Could you check a few things on this model? Use its own coordinates, in mm. A direction names the side the tool comes from. Round coordinates to 2 decimals unless told otherwise and drop trailing zeros. Loops run counter-clockwise (first coordinate to the right, second up) from the corner with the lowest first, then second, coordinate; pieces in that order, holes last. Notation, with made-up numbers: M 47.25,32.5 L 58.25,32.5 A16 cw 58.25,36.5 Z; hole C 28,54.5 d5. An arc over 180 degrees is marked long. One line per item, written item: value. Start each with the question number.
Q1. I'm going to push flat-ended pins straight in: pin 1 Ø1.8 at (y, z) = (24.5, 5.5) entering from -X; pin 2 Ø11 at (y, z) = (9.5, 107.5) entering from -X; pin 3 Ø5 at (x, z) = (19.5, 106.5) entering from +Y; pin 4 Ø6 at (x, y) = (23, -36.5) entering from +Z. Where does each tip first touch, or does it pass through?
Q2. Which directions (+Z, -Z, +X, -X, +Y, -Y) give clear straight access to the entire face, cutting with the end or side of a thin tool? Please do faces 4 (the face through (19.38, 23.7, 21.69)), 5 (the face through (3.711, -43.335, 14.252)), 6 (the face through (19.199, 19.981, 92.714)), 7 (the face through (28.813, 22, 52)), 8 (the face through (27.2, 19.51, 101.73)).
Q3. Imagine slicing it at A-A (y = 11.5). Please give me the cut outline in (x, z).
Q4. Please list where these lines run through material, in increasing order: line 1 along X through (y, z) = (-44, 18); line 2 along Z through (x, y) = (10.5, -24.5); line 3 along X through (y, z) = (23, 55.5).
Q5. Thinking about a two-plate mould opening in Y: for faces 1 (the face through (9.73, -39.325, 59.103)), 2 (the face through (9.763, 22, 50)), 3 (the face through (19.38, 23.97, 16.62)), which applies, released by +Y, released by -Y, zero draft, split by the parting line, or undercut?
Q6. Imagine slicing it at B-B (z = 29). Please give me the cut outline in (x, y), then the cut area to 3 significant figures.
Q7. Imagine slicing it at D-D (y = 0.5). Please give me the cut outline in (x, z).
Q8. Imagine slicing it at C-C (x = 2). Please give me the cut outline in (y, z).
from build123d import *

# Parameters (mm, degrees)
F0_W     = 63.5
F0_H     = 63.5
F1_DEPTH = 101.6
F1_TAPER = 3
F3_DEPTH = 10.16
F4_W     = 7.62
F4_H     = 7.62
F5_DEPTH = 7.62
F5_TAPER = 26
F7_DEPTH = 2.54
F8_W     = 12.7
F8_H     = 12.7
F9_DEPTH = 5.08


with BuildPart() as f1:
    # F0 (on Top) → F1 (new body)
    with BuildSketch(Plane.XY):
        with Locations((3.6575980484, -9.4182148212)):
            Rectangle(F0_W, F0_H)
    extrude(amount=F1_DEPTH, taper=F1_TAPER)

    # F2 (on face) → F3 (join)
    with BuildSketch(Plane.XY.offset(101.6)):
        Polygon((-12.6077715764, -15.5235844461), (-22.7677715764, -15.5235844461), (-22.7677715764, -35.8435844461), (-12.6077715764, -35.8435844461), (-2.4477715764, -35.8435844461), (-2.4477715764, -25.6835844461), (-12.6077715764, -25.6835844461), align=None)
        Polygon((19.9229676733, -35.8435844461), (30.0829676733, -35.8435844461), (30.0829676733, -15.5235844461), (19.9229676733, -15.5235844461), (19.9229676733, -25.6835844461), (9.7629676733, -25.6835844461), (9.7629676733, -35.8435844461), align=None)
        Polygon((-12.6077715764, 17.0071548036), (-22.7677715764, 17.0071548036), (-22.7677715764, -3.3128451964), (-12.6077715764, -3.3128451964), (-12.6077715764, 6.8471548036), (-2.4477715764, 6.8471548036), (-2.4477715764, 17.0071548036), align=None)
        Polygon((30.0829676733, -3.3128451964), (30.0829676733, 17.0071548036), (19.9229676733, 17.0071548036), (9.7629676733, 17.0071548036), (9.7629676733, 6.8471548036), (19.9229676733, 6.8471548036), (19.9229676733, -3.3128451964), align=None)
    extrude(amount=F3_DEPTH)

    # F4 (on face) → F5 (join)
    with BuildSketch(Plane(origin=(0, -41.0554529271, 2.1516251154), x_dir=(1, 0, 0), z_dir=(0, -0.9986295348, 0.0523359562))):
        with Locations((-19.2024019516, 14.3554221105)):
            Rectangle(F4_W, F4_H)
        with Locations((3.6575980484, 14.3554221105)):
            Rectangle(F4_W, F4_H)
        with Locations((26.5175980484, 14.3554221105)):
            Rectangle(F4_W, F4_H)
    extrude(amount=F5_DEPTH, taper=F5_TAPER)

    # F6 (on face) → F7 (join)
    with BuildSketch(Plane(origin=(0, -41.0554529271, 2.1516251154), x_dir=(1, 0, 0), z_dir=(0, -0.9986295348, 0.0523359562))):
        Polygon((-11.5824019516, 56.964216193), (-11.5824019516, 41.724216193), (18.8975980484, 41.724216193), (18.8975980484, 56.964216193), (18.8975980484, 62.044216193), (12.5475980484, 62.044216193), (12.5475980484, 56.964216193), (6.8325980484, 56.964216193), (6.8325980484, 62.044216193), (0.4825980484, 62.044216193), (0.4825980484, 56.964216193), (-5.2324019516, 56.964216193), (-5.2324019516, 62.044216193), (-11.5824019516, 62.044216193), align=None)
    extrude(amount=F7_DEPTH)

    # F8 (on face) → F9 (join)
    with BuildSketch(Plane(origin=(0, 22.2706172509, 1.1671535934), x_dir=(-1, 0, 0), z_dir=(0, 0.9986295348, 0.0523359562))):
        Polygon((-28.8129676733, 100.5706750214), (-28.8129676733, -1.1687553319), (-25.6379676733, -1.1687553319), (-25.6379676733, 15.3412446681), (-12.9379676733, 15.3412446681), (-12.9379676733, -1.1687553319), (-9.7629676733, -1.1687553319), (-9.7629676733, 100.5706750214), (-12.9379676733, 100.5706750214), (-12.9379676733, 91.5412446681), (-25.6379676733, 91.5412446681), (-25.6379676733, 100.5706750214), align=None)
        with Locations((-19.2879676733, 26.7712446681)):
            Rectangle(F8_W, F8_H, mode=Mode.SUBTRACT)
        with Locations((-19.2879676733, 44.5512446681)):
            Rectangle(F8_W, F8_H, mode=Mode.SUBTRACT)
        with Locations((-19.2879676733, 80.1112446681)):
            Rectangle(F8_W, F8_H, mode=Mode.SUBTRACT)
        with Locations((-19.2879676733, 62.3312446681)):
            Rectangle(F8_W, F8_H, mode=Mode.SUBTRACT)
    extrude(amount=F9_DEPTH)


solid = f1.part
Report:
1. pin 1: stops at x = 9.76
1. pin 2: stops at x = -22.77
1. pin 3: stops at y = 17.01
1. pin 4: stops at z = 111.76
2. face 4: none
2. face 5: +X, -X, -Y
2. face 6: +Z
2. face 7: +Z, +X, +Y
2. face 8: +Z, +X, -X
3. outline: M -28.09,0 L 35.41,0 L 30.08,101.6 L 30.08,111.76 L 9.76,111.76 L 9.76,101.6 L -2.45,101.6 L -2.45,111.76 L -22.77,111.76 L -22.77,101.6 Z
4. line 1: x = -21.17 to -17.23, 1.69 to 5.63, 24.55 to 28.49
4. line 2: z = 0 to 101.6
4. line 3: x = 9.76 to 28.81
5. face 1: undercut
5. face 2: zero draft
5. face 3: released by +Y
6. outline: M -26.57,-39.65 L 33.89,-39.65 L 33.89,20.81 L 28.81,20.81 L 28.81,25.9 L 25.64,25.9 L 25.64,20.81 L 12.94,20.81 L 12.94,25.9 L 9.76,25.9 L 9.76,20.81 L -26.57,20.81 Z
6. area: 3,690 mm²
7. outline: M -28.09,0 L 35.41,0 L 30.08,101.6 L 30.08,111.76 L 19.92,111.76 L 19.92,101.6 L -12.61,101.6 L -12.61,111.76 L -22.77,111.76 L -22.77,101.6 Z
8. outline: M -44.8,15.06 L -40.5,12.68 L -41.17,0 L 22.33,0 L 17.01,101.6 L -35.84,101.6 L -37.81,64.11 L -40.34,64.24 L -41.41,43.95 L -38.87,43.82 L -40.1,20.29 L -44.62,18.37 Z
